Geometry: see drawing. Coordinates: mm, zero at the bounding-box minimum. Give positions to 0.01 mm unless a question says otherwise; leave off trailing zeros. Loops run counter-clockwise (first coordinate to the right, second up) from the corner with the lowest first, then second, coordinate; pieces in that order, holes last. Notation, with made-up numbers: (-27.5, 1.25) -> (26.5, 1.25) arc R12 ccw to (26.5, 9.25) -> close; hole circle Ø2 at (78.5, -22). An arc over 180 degrees is marked (long way). Return JSON: item names as keys, results as strings. Group by question number.
(1) Cut plane B-B on x = 32.5. Return loops of the section in (y, z).
(2) Cut plane C-C on z = 1.9. Return loops of the section in (x, y).
(3) Ray query, line 1 (X direction, y = 10, z = 3.5); line 2 (Y direction, x = 7.5, z = 3.55). Return the intervals inside material, ascending. Write a range as from..to.
(4) Cut plane A-A on y = 10. Return loops of the section in (x, z).
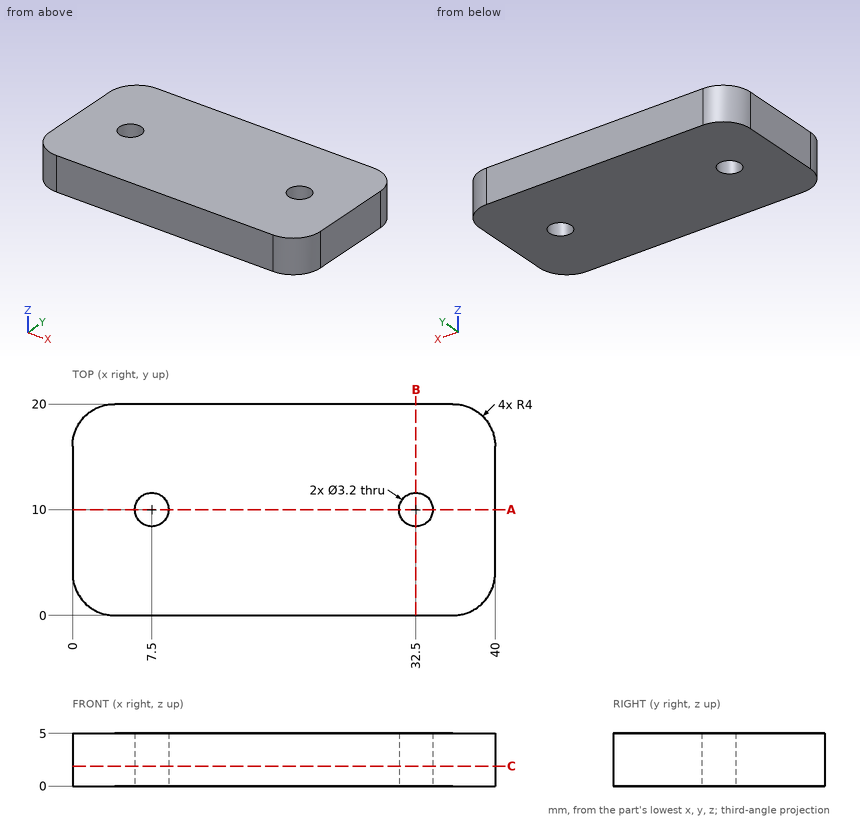
Answers:
{
 "1": {"outline": "(0, 0) -> (8.4, 0) -> (8.4, 5) -> (0, 5) -> close; (11.6, 0) -> (20, 0) -> (20, 5) -> (11.6, 5) -> close"},
 "2": {"outline": "(0, 4) arc R4 ccw to (4, 0) -> (36, 0) arc R4 ccw to (40, 4) -> (40, 16) arc R4 ccw to (36, 20) -> (4, 20) arc R4 ccw to (0, 16) -> close; hole circle Ø3.2 at (7.5, 10); hole circle Ø3.2 at (32.5, 10)"},
 "3": {"line 1": "0..5.9, 9.1..30.9, 34.1..40", "line 2": "0..8.4, 11.6..20"},
 "4": {"outline": "(0, 0) -> (5.9, 0) -> (5.9, 5) -> (0, 5) -> close; (9.1, 0) -> (30.9, 0) -> (30.9, 5) -> (9.1, 5) -> close; (34.1, 0) -> (40, 0) -> (40, 5) -> (34.1, 5) -> close"}
}
